Autodesk Inventor part; units mm, degrees
ref_plane "YZ Plane" through (0, 0, 0) normal (1, 0, 0) x (0, 1, 0)
ref_plane "XZ Plane" through (0, 0, 0) normal (0, 1, 0) x (-1, 0, 0)
ref_plane "XY Plane" through (0, 0, 0) normal (0, 0, 1) x (1, 0, 0)
sketch "Sketch1" plane through (0, 0, 0) normal (1, 0, 0) x (0, 1, 0)
  line L0 (0, 55.88) -> (914.4, 55.88)
  arc A0 (914.4, 0) -> (914.4, 55.88) centre (914.4, 27.94) ccw
  line L1 (914.4, 0) -> (0, 0)
  line L2 (0, 56.134) -> (914.4, 56.134)
  arc A1 (914.4, -0.254) -> (914.4, 56.134) centre (914.4, 27.94) ccw
  line L3 (914.4, -0.254) -> (0, -0.254)
  line L4 (0, 55.88) -> (0, 56.134)
  line L5 (0, -0.254) -> (0, 0)
  dimension "d6" = 27.94
  dimension "d7" = 914.4
  dimension "d12" = 0.254
extrude "Extrusion2" add sketch "Sketch1" against normal blind 25.4
properties part number "guide"
Could you check a few things on this model? Use its own coordinates, in mm. Give positions to 0.01 mm unless a question says otherwise; leave off trailing zeros. Order: outer loops, then holes, each group sorted by start corner. A loop starts at its lowest first (then second) coordinate and runs counter-clockwise, first axis right, second up. Notation, with made-up numbers: (47.25, 23) - (99.25, 23) arc R20 ccw to (99.25, 37) - close; hole circle Ø7 at (38.5, 22). An arc over 180 degrees is marked (long way). One line per question, with ' | ' between items. Start each with the question number.
Item 1: I want a section at C-C on z = 27.94. Write out the boundary of the cut face in (x, y).
Item 2: I need wall thicknesses on probe 1 along Z at (x, y) = (-22.25, 675); probe 2 along Y at (x, z) = (-2.75, 27); probe 3 along Y at (x, z) = (-6.75, 7). Which ranges of each line are inside material? Lowest first, please. Write a range as [from, to].
Item 3: I want a section at A-A on y = 162. Write out the boundary of the cut face in (x, z).
Item 4: I'm going to push flat-ended pins straight in: pin 1 Ø1 at (x, z) = (-21.5, 31) entering from -Y; pin 2 Ø1.5 at (x, z) = (-12.5, 50) entering from +Y; pin 3 Ø8 at (x, z) = (-12, 49) entering from -Y. Where does each tip first touch, or does it pass through?
Item 5: I want a section at B-B on x = -12.5. Write out the boundary of the cut face in (y, z), then the cut area to 3 significant figures.
Item 6: Thinking about a two-plate mould opening in Z: for faces 1 (the flat face through (-13, 464, -0.254)), 2 (the cylindrical face through (-12.522, 942.587, 27.32)), 3 (the cylindrical face through (-12.522, 942.333, 27.326)), 4 (the flat face through (-13, 451, 56.134)), which applies, pulls with the +Z half, pulls with the -Z half, needs draft (parallel to the pull), parting line crosses it, or undercut?
Verdict:
1) outline: (-25.4, 942.34) - (0, 942.34) - (0, 942.59) - (-25.4, 942.59) - close
2) probe 1: [-0.25, 0], [55.88, 56.13] | probe 2: [942.32, 942.58] | probe 3: [932.9, 933.28]
3) outline: (-25.4, -0.25) - (0, -0.25) - (0, 0) - (-25.4, 0) - close; (-25.4, 55.88) - (0, 55.88) - (0, 56.13) - (-25.4, 56.13) - close
4) pin 1: y = 942.11 | pin 2: y = 932.86 | pin 3: y = 926.75
5) outline: (0, -0.25) - (914.4, -0.25) arc R28.19 ccw to (914.4, 56.13) - (0, 56.13) - (0, 55.88) - (914.4, 55.88) arc R27.94 cw to (914.4, 0) - (0, 0) - close | area: 487 mm^2
6) face 1: pulls with the -Z half | face 2: parting line crosses it | face 3: undercut | face 4: pulls with the +Z half
